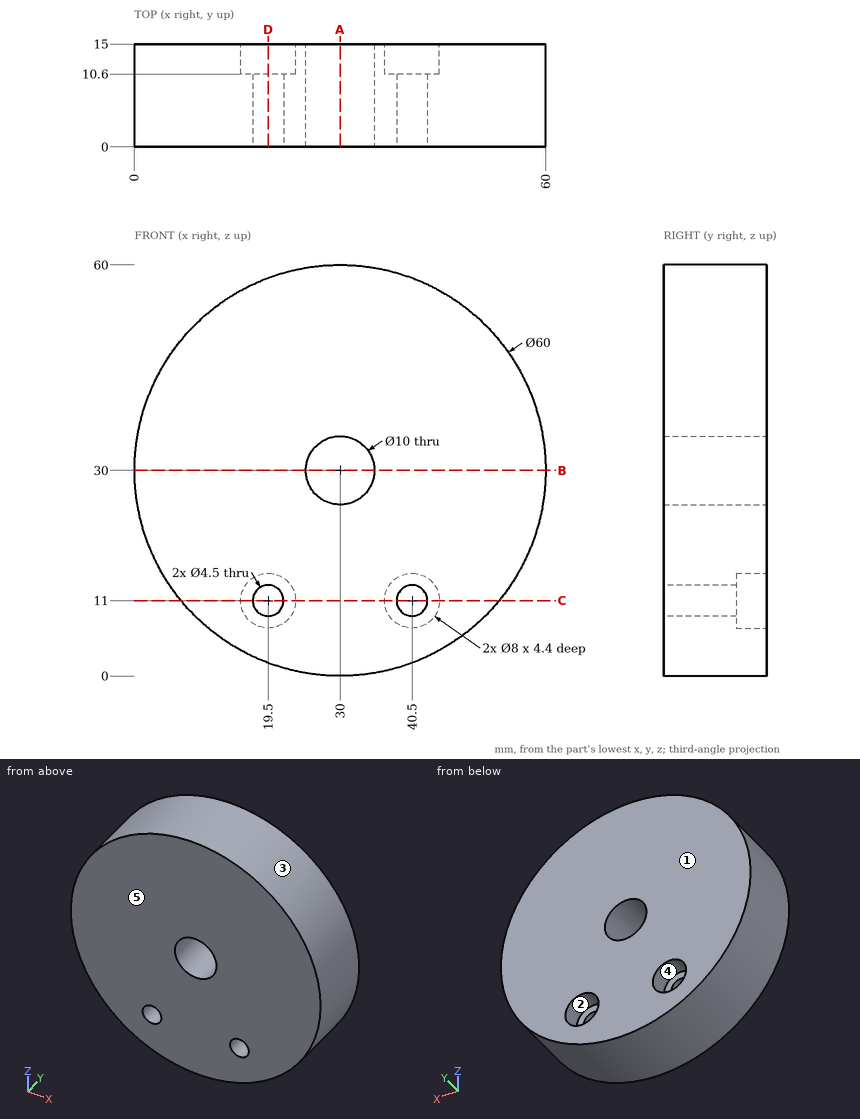
Study the drawing (mm; zero at the part's minimum x, y, z) and answer. A direction names the side the tool comes from. Give positions to 0.01 mm unless a question says otherwise; leave off trailing zeros. Write each loop counter-clockwise with the first axis right and the second up, starting at its lowest first coordinate (ties: lowest second). Pieces come first, ordered by that corner, then holes. Notation, with made-up numbers: (83, -22.75) -> (124, -22.75) arc R30 ccw to (124, 15.25) -> close; hole circle Ø10 at (26.5, 15). An arc over 180 degrees is marked (long way). Answer as a JSON object with one key per item and string values. Group by question number.
1) Find section A-A (x = 30). Write down the section's boundary in (y, z), and give its area (3 significant figures).
2) Find section B-B (z = 30). Write down the section's boundary in (x, y).
3) Find section C-C (z = 11). Write down the section's boundary in (x, y).
4) Find section D-D (x = 19.5). Write down the section's boundary in (y, z).
5) Each of these flat-tipped pins is pushed along its axis until it touches: P1, Ø6, axis at x = 39.5, y = 8, coming from the +Z side; P2, Ø6.5, axis at x = 41, z = 12, coming from the +Y side; P3, Ø6, axis at x = 22, y = 11.5, coming from the +Z side; P4, Ø6, axis at y = 13, z = 49, coming from the -X side. Where does it stop, or does it pass through?
6) The mould has two halves that part along X. Classify the marked faces 1, 2 and 3: +X half, -X half, draft (parallel to the pull), parting line (faces both ways), or undercut.
7) A tool of negligible diameter and unlimited length cuts with its end or side. For the marked faces 4 and 5, from which of +Z, -Z, +X, -X, +Y, -Y can it reach the whole face along a straight path? Write none if from no direction.
8) Consider L1, parallel to Z at x = 30, y = 4.5; L2, parallel to X at y = 3.75, z = 11; L3, parallel to X at y = 12.25, z = 11. Determine where each line is inside the solid, lowest interval first. Write a range as from..to.
Values follow:
{
 "1": {"outline": "(0, 0) -> (15, 0) -> (15, 25) -> (0, 25) -> close; (0, 35) -> (15, 35) -> (15, 60) -> (0, 60) -> close", "area": "750 mm2"},
 "2": {"outline": "(0, 0) -> (25, 0) -> (25, 15) -> (0, 15) -> close; (35, 0) -> (60, 0) -> (60, 15) -> (35, 15) -> close"},
 "3": {"outline": "(6.78, 0) -> (17.25, 0) -> (17.25, 10.6) -> (15.5, 10.6) -> (15.5, 15) -> (6.78, 15) -> close; (21.75, 0) -> (38.25, 0) -> (38.25, 10.6) -> (36.5, 10.6) -> (36.5, 15) -> (23.5, 15) -> (23.5, 10.6) -> (21.75, 10.6) -> close; (42.75, 0) -> (53.22, 0) -> (53.22, 15) -> (44.5, 15) -> (44.5, 10.6) -> (42.75, 10.6) -> close"},
 "4": {"outline": "(0, 1.9) -> (15, 1.9) -> (15, 7) -> (10.6, 7) -> (10.6, 8.75) -> (0, 8.75) -> close; (0, 13.25) -> (10.6, 13.25) -> (10.6, 15) -> (15, 15) -> (15, 58.1) -> (0, 58.1) -> close"},
 "5": {"P1": "stops at z = 59.29", "P2": "stops at y = 15", "P3": "stops at z = 59.58", "P4": "stops at x = 4.62"},
 "6": {"face 1": "draft", "face 2": "undercut", "face 3": "parting line"},
 "7": {"face 4": "+Y", "face 5": "+Z, -Z, +X, -X, -Y"},
 "8": {"L1": "z = 0..25, 35..60", "L2": "x = 6.78..17.25, 21.75..38.25, 42.75..53.22", "L3": "x = 6.78..15.5, 23.5..36.5, 44.5..53.22"}
}
